from build123d import *

# Parameters (mm, degrees)
F0_W     = 85
F0_H     = 19.05
F0_R     = 1.6
F0_R_2   = 5
F1_DEPTH = 6.35
F2_R     = 1.5
F3_DEPTH = 5
F4_R     = 3


with BuildPart() as f1:
    # F0 (on Front) → F1 (new body)
    with BuildSketch(Plane.XZ):
        Rectangle(F0_W, F0_H)
        with Locations((-15.5, 0)):
            Circle(F0_R, mode=Mode.SUBTRACT)
        with Locations((32.5, 0)):
            Circle(F0_R_2, mode=Mode.SUBTRACT)
    extrude(amount=F1_DEPTH)

    # F2 (on face) → F3 (cut)
    with BuildSketch(Plane(origin=(0, 0, -9.525), x_dir=(1, 0, 0), z_dir=(0, 0, -1))):
        with Locations((-25.5, 3.175)):
            Circle(F2_R)
        with Locations((25.5, 3.175)):
            Circle(F2_R)
    extrude(amount=-F3_DEPTH, mode=Mode.SUBTRACT)

    # F4
    f4_edges = [f1.edges().sort_by_distance(p)[0] for p in [
        (42.5, -3.175, 9.525),
        (42.5, -3.175, -9.525),
        (-42.5, -3.175, -9.525),
        (-42.5, -3.175, 9.525),
    ]]
    fillet(f4_edges, radius=F4_R)


solid = f1.part
Can you work these out from the model? Positions are in its coordinate system, mm. A direction names the side the tool comes from. Round coordinates to 2 decimals unless told otherwise and drop trailing zeros. Order: outer loops, then holes, each group sorted by start corner. A loop starts at its lowest first (then second) coordinate and runs counter-clockwise, first axis right, second up. Notation, with made-up numbers: (85.25, -7.5) -> (89.25, -7.5) arc R22 ccw to (89.25, 31.5) -> close; hole circle Ø2 at (27, 39). An arc over 180 degrees is marked (long way). Write each question's results on one line, items separated by ' | '. Start each with the question number.
Item 1: Thinking about a two-plate mould opening in X: for faces 3 (the cylindrical face through (-41.645, -3.219, -8.623)), 4 (the flat face through (25, -3, -4.525)), 5 (the flat face through (42.5, -3, 0)), which applies, +X half, -X half, draft (parallel to the pull), parting line (faces both ways), or undercut?
Item 2: Please list where these lines run through material, in increasing order: L1, parallel to Z at x = -15.5, y = -2.25 (3 decimals); L2, parallel to X at y = -1, z = -0.5; L3, parallel to X at y = -2.25, z = -7.5.
Item 3: If we section it at D-D, the plane z = 3.5: Write out the boundary of the cut face in (x, y), then the cut area to 3 significant figures.
Item 4: If we section it at C-C, the plane y = -5.5: Write out the boundary of the cut face in (x, z) (3 decimals), then the cut area to 3 significant figures.
Item 5: If we section it at B-B, the plane z = 0: Write out the boundary of the cut face in (x, y), then the cut area to 3 significant figures.
Item 6: Which directions (+Z, -Z, +X, -X, +Y, -Y) give clear straight access to the entire face, cutting with the end or side of a thin tool? Please do faces 1 (the cylindrical face through (24, -3.2, -7.1)), 2 (the flat face through (-42.5, -3, 0)).
Item 7: Will this pin go through, and if not, where does the flat tip stop? pin 1 (2.5 mm diameter, centred on x = -25.5, y = -3.175, fed in from -Z) (3 decimals).
Item 8: If we section it at A-A, the plane x = 32.5: Write out the boundary of the cut face in (y, z) (3 decimals).
Results:
1) face 3: -X half | face 4: undercut | face 5: +X half
2) L1: z = -9.525 to -1.6, 1.6 to 9.525 | L2: x = -42.5 to -17.02, -13.98 to 27.53, 37.47 to 42.5 | L3: x = -42.34 to -26.68, -24.32 to 24.32, 26.68 to 42.34
3) outline: (-42.5, -6.35) -> (28.93, -6.35) -> (28.93, 0) -> (-42.5, 0) -> close; (36.07, -6.35) -> (42.5, -6.35) -> (42.5, 0) -> (36.07, 0) -> close | area: 494 mm2
4) outline: (-42.5, -6.525) arc R3 ccw to (-39.5, -9.525) -> (39.5, -9.525) arc R3 ccw to (42.5, -6.525) -> (42.5, 6.525) arc R3 ccw to (39.5, 9.525) -> (-39.5, 9.525) arc R3 ccw to (-42.5, 6.525) -> close; hole circle Ø3.2 at (-15.5, 0); hole circle Ø10 at (32.5, 0) | area: 1,520 mm2
5) outline: (-42.5, -6.35) -> (-17.1, -6.35) -> (-17.1, 0) -> (-42.5, 0) -> close; (-13.9, -6.35) -> (27.5, -6.35) -> (27.5, 0) -> (-13.9, 0) -> close; (37.5, -6.35) -> (42.5, -6.35) -> (42.5, 0) -> (37.5, 0) -> close | area: 456 mm2
6) face 1: -Z | face 2: +Z, -Z, -X, +Y, -Y
7) pin 1: stops at z = -4.525
8) outline: (-6.35, -9.525) -> (0, -9.525) -> (0, -5) -> (-6.35, -5) -> close; (-6.35, 5) -> (0, 5) -> (0, 9.525) -> (-6.35, 9.525) -> close
